Geometry check sheet. Reference: the model listing, model coordinates, mm. Face numbers are marked on the shaded views. Give positions to 0.01 mm unless a question says otherwise; leave off trailing zeros. Write each loop counter-clockwise with the first axis right and the second up, starting at its lowest first coordinate (ties: lowest second). Pieces come first, ordered by that corner, then holes. Notation, with made-up numbers: (43, 88.5) -> (87, 88.5) arc R16 cw to (87, 107.5) -> close; hole circle Ø3 at (62, -22). An arc over 180 degrees is marked (long way). One line per item, written item: value.
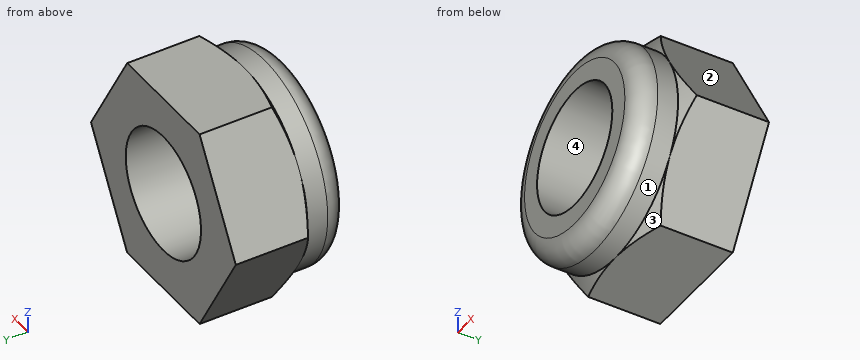
from build123d import *

# Parameters (mm, degrees)
F0_R     = 3
F1_DEPTH = 4
F4_R     = 5
F4_R_2   = 3
F5_DEPTH = 2
F6_R     = 1


with BuildPart() as f1:
    # F0 (on Front) → F1 (new body)
    with BuildSketch(Plane.XZ):
        Polygon((2.886751, -5), (5.773503, 0), (2.886751, 5), (-2.886751, 5), (-5.773503, 0), (-2.886751, -5), align=None)
        Circle(F0_R, mode=Mode.SUBTRACT)
    extrude(amount=F1_DEPTH)

    # F2 (on Right) → F3 (revolve, cut)
    with BuildSketch(Plane.YZ):
        Polygon((-5.443376, 7.5), (-5.443376, 2.5), (-2.556624, 7.5), align=None)
    revolve(axis=Axis((0, 0, 0), (0, 1, 0)), mode=Mode.SUBTRACT)

    # F4 (on face) → F5 (join)
    with BuildSketch(Plane.XZ.offset(4)):
        Circle(F4_R)
        Circle(F4_R_2, mode=Mode.SUBTRACT)
    extrude(amount=F5_DEPTH)

    # F6
    f6_edges = [f1.edges().sort_by_distance(p)[0] for p in [
        (-5, -6, 0),
    ]]
    fillet(f6_edges, radius=F6_R)


solid = f1.part
1) Depth check by flat-ended pin: pin 1 Ø1 at (x, y) = (2, -5.5) entering from -Z; pin 2 Ø2 at (y, z) = (-2.5, 2) entering from -X. Enter the tip coordinate at first touch or a pass-through.
Verdict:
pin 1: z = -4.72
pin 2: x = -5.2
2) Sectioned sample at A-A on y = -1.75. Record the cut outline in (x, z), plus the area to 3 significant figures.
Verdict:
outline: (-5.77, 0) -> (-2.89, -5) -> (2.89, -5) -> (5.77, 0) -> (2.89, 5) -> (-2.89, 5) -> close; hole circle Ø6 at (0, 0)
area: 58.3 mm^2
3) Sectioned sample at B-B on y = -5.3. Record the cut outline in (x, z).
Verdict:
outline: circle Ø9.91 at (0, 0); hole circle Ø6 at (0, 0)
4) Mould release check, pull along Z, two halves, no side actions. Record for the marked faces 1, 2, 3 and 4: released by +Z, released by -Z, zero draft, split by the parting line, or undercut.
Verdict:
face 1: split by the parting line
face 2: released by +Z
face 3: released by -Z
face 4: undercut
5) Scan lines: probe 1 along Z at (x, y) = (0, -3.25); probe 2 along Z at (x, y) = (-2.75, -1.9); probe 3 along Z at (x, y) = (4, -4.7). Record each from-to range of solid material in increasing order.
Verdict:
probe 1: -5 to -3, 3 to 5
probe 2: -5 to -1.2, 1.2 to 5
probe 3: -3 to 3
